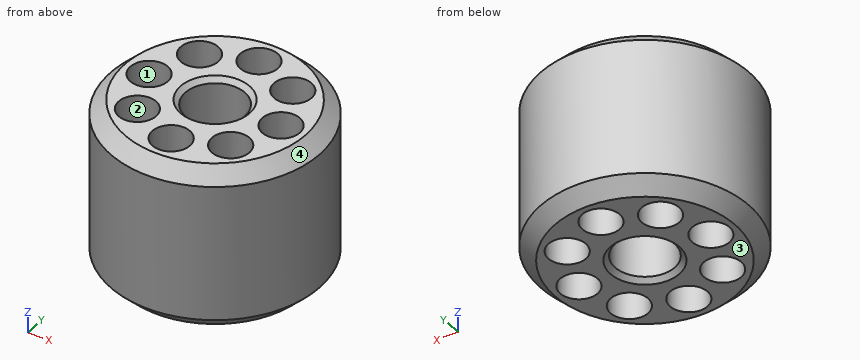
```python
from build123d import *

# Parameters (mm, degrees)
F0_R     = 22.225
F0_R_2   = 4
F0_R_3   = 6.35
F1_DEPTH = 35
F2_SIZE  = 3
F3_SIZE  = 1


with BuildPart() as f1:
    # F0 (on Top) → F1 (new body)
    with BuildSketch(Plane.XY):
        Circle(F0_R)
        with Locations((-9.899495, -9.899495)):
            Circle(F0_R_2, mode=Mode.SUBTRACT)
        with Locations((0, -14)):
            Circle(F0_R_2, mode=Mode.SUBTRACT)
        with Locations((9.899495, -9.899495)):
            Circle(F0_R_2, mode=Mode.SUBTRACT)
        with Locations((-14, 0)):
            Circle(F0_R_2, mode=Mode.SUBTRACT)
        with Locations((-9.899495, 9.899495)):
            Circle(F0_R_2, mode=Mode.SUBTRACT)
        Circle(F0_R_3, mode=Mode.SUBTRACT)
        with Locations((9.899495, 9.899495)):
            Circle(F0_R_2, mode=Mode.SUBTRACT)
        with Locations((14, 0)):
            Circle(F0_R_2, mode=Mode.SUBTRACT)
        with Locations((0, 14)):
            Circle(F0_R_2, mode=Mode.SUBTRACT)
    extrude(amount=F1_DEPTH)

    # F2
    f2_edges = [f1.edges().sort_by_distance(p)[0] for p in [
        (-22.225, 0, 35),
        (-22.225, 0, 0),
    ]]
    chamfer(f2_edges, length=F2_SIZE)

    # F3
    f3_edges = [f1.edges().sort_by_distance(p)[0] for p in [
        (-6.35, 0, 0),
        (-6.35, 0, 35),
    ]]
    chamfer(f3_edges, length=F3_SIZE)


solid = f1.part
```
Input: part model. Units: mm. Frame: model coordinates. Face numbers are marked on the shaded views. Coordinates: 2 decimals unless noted, no trailing zeros. Loops run counter-clockwise (first coordinate to the right, second up) from the corner with the lowest first, then second, coordinate; pieces in that order, holes last. Notation, with made-up numbers: (-33.5, 18) - (-22.5, 18) arc R31 cw to (-22.5, 47) - close; hole circle Ø9 at (85, 14.5). An arc over 180 degrees is marked (long way). Answer in a Markdown table with one row per item.
(1) Cut plane A-A on y = 0. Output: boundary loops of the cut face in (x, z) (3 decimals), plus the area to 3 significant figures.
Model answer:
| item | result |
|---|---|
| outline | (-22.225, 3) - (-19.225, 0) - (-18, 0) - (-18, 35) - (-19.225, 35) - (-22.225, 32) - close; (-10, 0) - (-7.35, 0) - (-6.35, 1) - (-6.35, 34) - (-7.35, 35) - (-10, 35) - close; (6.35, 1) - (7.35, 0) - (10, 0) - (10, 35) - (7.35, 35) - (6.35, 34) - close; (18, 0) - (19.225, 0) - (22.225, 3) - (22.225, 32) - (19.225, 35) - (18, 35) - close |
| area | 531 mm² |
(2) Pin query (flat end, axial travel): P1, Ø9, axis at x = 14, y = 0, coming from the +Z side; P2, Ø6.5, axis at x = 0, y = 14, coming from the -Z side; P3, Ø1, axis at y = 4, z = 23, coming from the -X side; P4, Ø3, axis at y = -8.5, z = 5.5, coming from the -X side. Return the tip coordinate at first contact, or that it passes through.
Model answer:
| item | result |
|---|---|
| P1 | stops at z = 35 |
| P2 | passes through |
| P3 | stops at x = -21.95 |
| P4 | stops at x = -21.09 |
(3) Material intervals for L1, parallel to Y at x = 0, z = 23 (3 decimals); L2, parallel to Y at x = 1.5, z = 13.5; L3, parallel to X at y = -13, z = 30, sorted ascending. Write a range as from..to.
Model answer:
| item | result |
|---|---|
| L1 | y = -22.225..-18, -10..-6.35, 6.35..10, 18..22.225 |
| L2 | y = -22.17..-17.71, -10.29..-6.17, 6.17..10.29, 17.71..22.17 |
| L3 | x = -18.03..-12.43, -7.37..-3.87, 3.87..7.37, 12.43..18.03 |
(4) Cut plane C-C on z = 21. Count the separate pieces of the cut face and the enclosed holes in it, plus the area to 3 significant figures.
Model answer:
| item | result |
|---|---|
| separate pieces | 1 |
| enclosed holes | 9 |
| area | 1,020 mm² |
(5) Mould query, pull axis X, two halves, no side actions, for the marked faces 1, 2, 3 and 4. Classes: pulls with the +X half, pulls with the -X half, needs draft (parallel to the pull), parting line crosses it, or undercut.
Model answer:
| item | result |
|---|---|
| face 1 | undercut |
| face 2 | undercut |
| face 3 | needs draft |
| face 4 | parting line crosses it |
